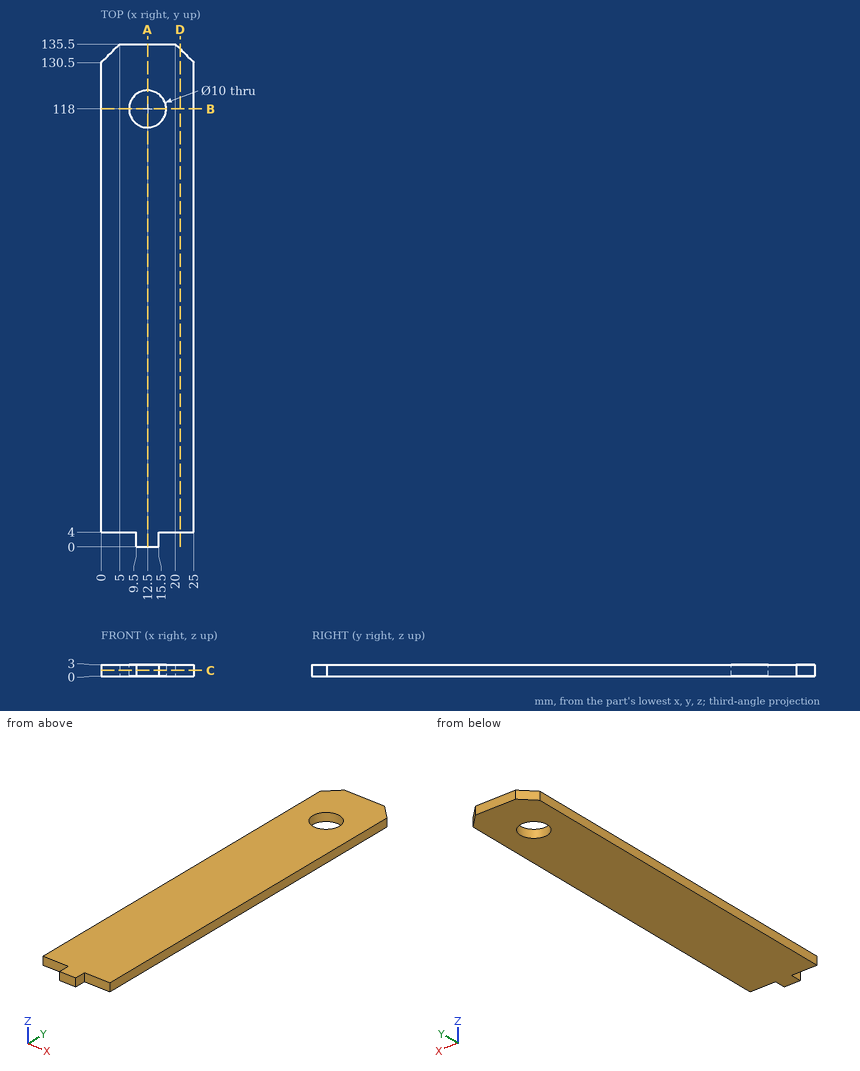
Job drawing, mm, ordinate dimensions from the low corner. One solid piece. Coordinates: 2 decimals unless noted, no trailing zeros. Order: outer loops, then holes, each group sorted by start corner. A loop starts at its lowest first (then second) coordinate and runs counter-clockwise, first axis right, second up. Notation, with made-up numbers: (60.5, -6) -> (109.5, -6) arc R18 ccw to (109.5, 21) -> close; hole circle Ø9 at (-11, 1.25). An arc over 180 degrees is marked (long way). Answer in a Markdown table with one row per item. Add a question column.
Q1. Band-saw the part on D-D, the plane x = 21.25. List the corners of the cut face in (y, z).
Q2. Band-saw the part on B-B, the plane y = 118. List the corners of the cut face in (x, z), then the cut area to 3 significant figures.
Q3. Band-saw the part on C-C, the plane z = 1.5. List the corners of the cut face in (x, y).
Q4. Drop a flat-ended pin along its axis: pin 1 (1.5 mm diameter, centred on x = 18.5, y = 75.5, fed in from -Z). Give the stop position or say it passes through.
Q5. Wall check: line 1 along Y through (x, z) = (12.5, 0.7); line 2 along X through (y, z) = (115, 1.95); line 3 along Y through (x, z) = (18.75, 2.05). Give the ranges that are in metal, low to high. Write a range as [from, to].
Q6. Band-saw the part on A-A, the plane x = 12.5. List the corners of the cut face in (y, z), then the cut area to 4 significant figures.
Answers follow:
| question | item | result |
|---|---|---|
| 1 | outline | (4, 0) -> (134.25, 0) -> (134.25, 3) -> (4, 3) -> close |
| 2 | outline | (0, 0) -> (7.5, 0) -> (7.5, 3) -> (0, 3) -> close; (17.5, 0) -> (25, 0) -> (25, 3) -> (17.5, 3) -> close |
| 2 | area | 45.0 mm^2 |
| 3 | outline | (0, 4) -> (9.5, 4) -> (9.5, 0) -> (15.5, 0) -> (15.5, 4) -> (25, 4) -> (25, 130.5) -> (20, 135.5) -> (5, 135.5) -> (0, 130.5) -> close; hole circle Ø10 at (12.5, 118) |
| 4 | pin 1 | z = 0 |
| 5 | line 1 | [0, 113], [123, 135.5] |
| 5 | line 2 | [0, 8.5], [16.5, 25] |
| 5 | line 3 | [4, 135.5] |
| 6 | outline | (0, 0) -> (113, 0) -> (113, 3) -> (0, 3) -> close; (123, 0) -> (135.5, 0) -> (135.5, 3) -> (123, 3) -> close |
| 6 | area | 376.5 mm^2 |
